Geometry: final body of the model. Coordinates: model frame, mm. Face numbers are marked on the shaded views. A direction names the side the tool comes from. Round coordinates to 2 decimals unless told otherwise and drop trailing zeros. Order: outer loops, then holes, each group sorted by start corner. A loop starts at its lowest first (then second) coordinate and runs counter-clockwise, first axis right, second up. Notation, with made-up numbers: (-8, -12) - (14, -12) arc R7 cw to (14, -3) - close; hole circle Ø7 at (76, 9.25). An arc over 180 degrees is marked (long way). Put each result on its own line as item: value. Start each with the question number.
(1) Section C-C (y = 1.5). Output: boundary loops of the cut face in (x, z), and give its area (3 significant figures).
(2) Pin query (flat end, axial travel): P1, Ø14.5, axis at x = -3.5, z = 7, coming from the +Y side; P2, Ø2, axis at y = -6, z = -3.5, coming from the -X side; P3, Ø8, axis at y = -7, z = -7.5, coming from the -X side. Return the tip coordinate at first contact, or that it passes through.
(3) Section D-D (x = 29). Output: boundary loops of the cut face in (y, z).
(4) Section A-A (z = 0). Output: boundary loops of the cut face in (x, y), and give its area (3 significant figures).
(5) Access query for the marked faces 5 and 6. Directions: +Z, -Z, +X, -X, +Y, -Y. A direction counts if a zero-diameter tool reaches every point of the face in a straight line with its end or side. Return the directions, or none.
(6) Material intervals for L1, parallel to X at y = 6, z = 7; L2, parallel to Y at x = 1, z = 4; L3, parallel to X at y = 1.25, z = 12, sorted ascending. Write a range as [from, to].
(7) Pull-direction query (X, two-part tool) for the marked faces 1, 2, 3 and 4; classes: released by +X, released by -X, zero draft, split by the parting line, or undercut.
(8) Section B-B (z = 5). Output: boundary loops of the cut face in (x, y).
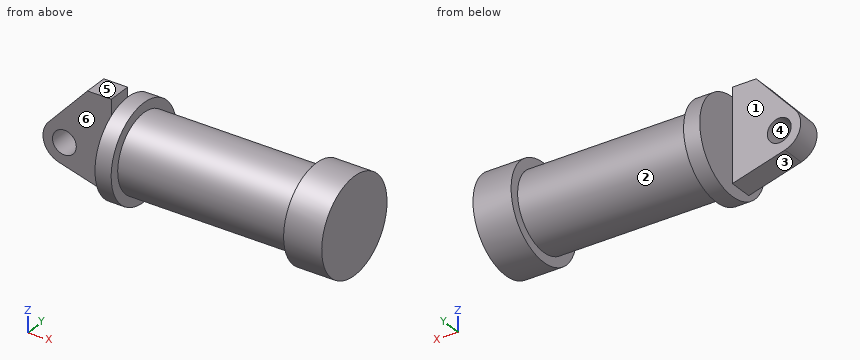
from build123d import *

# Parameters (mm, degrees)
F0_W     = 5.842
F0_H     = 12.7
F0_R     = 3.175
F2_DEPTH = 6.35


with BuildPart() as f1:
    # F0 (on Front) → F1 (revolve)
    with BuildSketch(Plane.XZ):
        Polygon((5.842, 12.7), (5.842, 0), (66.294, 0), (66.294, 12.7), (56.134, 12.7), (56.134, 10.16), (10.16, 10.16), (10.16, 12.7), align=None)
    revolve(axis=Axis((33.147, 0, 0), (-1, 0, 0)))

    # F0 (on Front) → F2 (join)
    with BuildSketch(Plane.XZ):
        with BuildLine():
            Line((-0.9398, 0), (0, 0))
            Line((0, 0), (0, 12.7))
            Line((0, 12.7), (5.842, 12.7))
            Line((5.842, 12.7), (5.842, 15.24))
            Line((5.842, 15.24), (-0.508, 15.24))
            Line((-0.508, 15.24), (-10.88063, 3.847543))
            ThreePointArc((-10.88063, 3.847543), (-4.591961, 5.329721), (-0.9398, 0))
        make_face()
        with Locations((2.921, 6.35)):
            Rectangle(F0_W, F0_H)
        with BuildLine():
            Line((5.842, 0), (0, 0))
            Line((0, 0), (-0.9398, 0))
            ThreePointArc((-0.9398, 0), (-3.195791, -4.549339), (-8.182663, -5.506983))
            Line((-8.182663, -5.506983), (5.842, -9.398))
            Line((5.842, -9.398), (5.842, 0))
        make_face()
        with BuildLine():
            ThreePointArc((-8.182663, -5.506983), (-3.195791, -4.549339), (-0.9398, 0))
            ThreePointArc((-0.9398, 0), (-4.591961, 5.329721), (-10.88063, 3.847543))
            ThreePointArc((-10.88063, 3.847543), (-12.145978, -1.583727), (-8.182663, -5.506983))
        make_face()
        with Locations((-6.6548, 0)):
            Circle(F0_R, mode=Mode.SUBTRACT)
    extrude(amount=F2_DEPTH)


solid = f1.part
Checks:
1. outline: (5.84, -12.61) - (10.16, -12.61) - (10.16, -10.05) - (56.13, -10.05) - (56.13, -12.61) - (66.29, -12.61) - (66.29, 12.61) - (56.13, 12.61) - (56.13, 10.05) - (10.16, 10.05) - (10.16, 12.61) - (5.84, 12.61) - close
1. area: 1,290 mm²
2. P1: stops at y = 0
2. P2: stops at x = -11.79
2. P3: stops at x = -11.13
3. outline: circle Ø20.32 at (0, 0)
4. outline: (-12.37, -6.35) - (-9.83, -6.35) - (-9.83, 0) - (-12.37, 0) - close; (-3.48, -6.35) - (5.84, -6.35) - (5.84, -12.7) - (10.16, -12.7) - (10.16, -10.16) - (56.13, -10.16) - (56.13, -12.7) - (66.29, -12.7) - (66.29, 12.7) - (56.13, 12.7) - (56.13, 10.16) - (10.16, 10.16) - (10.16, 12.7) - (5.84, 12.7) - (5.84, 0) - (-3.48, 0) - close
4. area: 1,380 mm²
5. face 5: +Z, +X, -X, +Y, -Y
5. face 6: +Z, -Z, -X, -Y
6. L1: x = [5.84, 66.29]
6. L2: y = [-6.35, 0]
6. L3: x = [5.84, 10.16], [56.13, 66.29]
7. face 1: zero draft
7. face 2: undercut
7. face 3: released by -X
7. face 4: undercut
8. outline: (-9.83, -6.35) - (5.84, -6.35) - (5.84, -11.67) - (10.16, -11.67) - (10.16, -8.84) - (56.13, -8.84) - (56.13, -11.67) - (66.29, -11.67) - (66.29, 11.67) - (56.13, 11.67) - (56.13, 8.84) - (10.16, 8.84) - (10.16, 11.67) - (5.84, 11.67) - (5.84, 0) - (-9.83, 0) - close
